Answer from the drawing. Dimensions are ordinates in mm from the lowest x, y and z of the part. A direction names the side the tool comes from. Coordinates: 2 decimals unless noted, no trailing zeros. Write each loop counter-clockwise with the first axis right and the second up, starting at its lowest first coordinate (ties: lowest second). Pieces come first, ordered by that corner, then holes. Notation, with made-up numbers: (-40, 19) - (-23, 19) arc R24 cw to (-23, 53) - close; hole circle Ø10 at (82.5, -30). An arc over 180 degrees is marked (long way). Return JSON: item names as keys, results as strings.
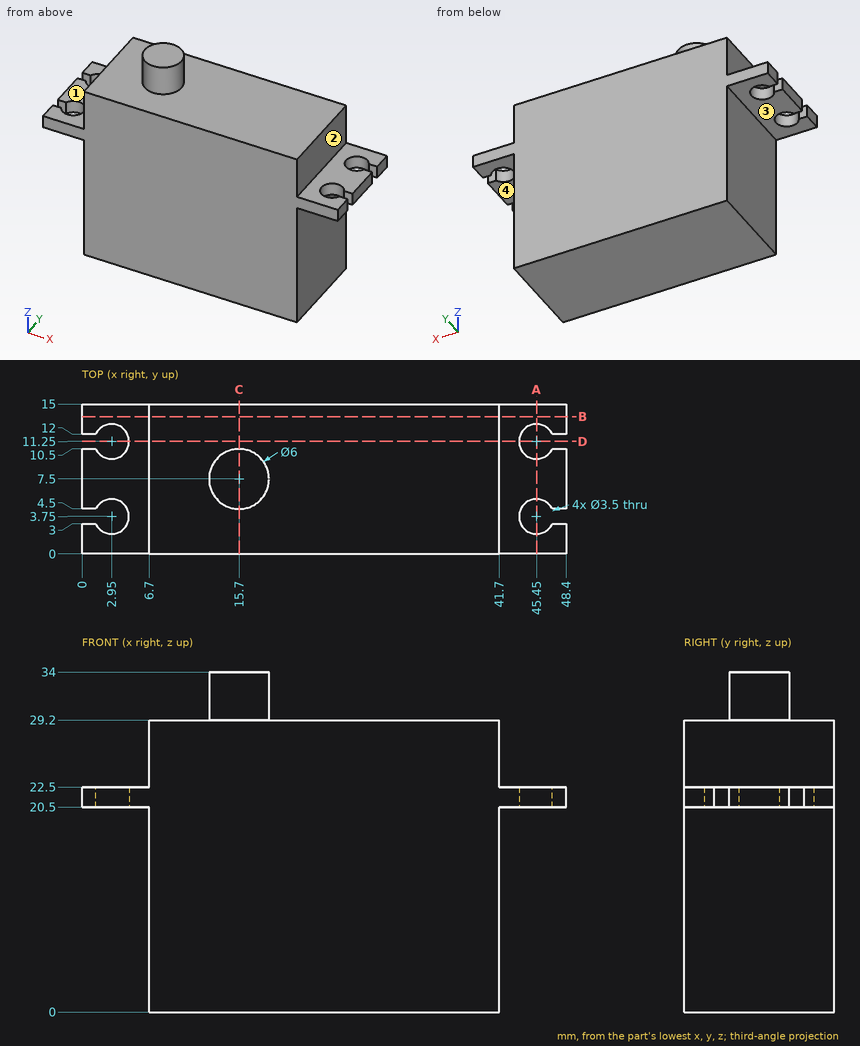
(1) A cutting plane is placed at D-D (y = 11.25). Determine the outline of the cut face in (x, z).
Answer:
{"outline": "(4.7, 20.5) - (6.7, 20.5) - (6.7, 0) - (41.7, 0) - (41.7, 20.5) - (43.7, 20.5) - (43.7, 22.5) - (41.7, 22.5) - (41.7, 29.2) - (6.7, 29.2) - (6.7, 22.5) - (4.7, 22.5) - close"}
(2) A cutting plane is placed at C-C (x = 15.7). Determine the outline of the cut face in (y, z).
Answer:
{"outline": "(0, 0) - (15, 0) - (15, 29.2) - (10.5, 29.2) - (10.5, 34) - (4.5, 34) - (4.5, 29.2) - (0, 29.2) - close"}
(3) Straight lines are drawn through the part: line 1 (Y direction, x = 2.95, z = 21.9); line 2 (Y direction, x = 45, z = 21); line 3 (Z direction, x = 43, y = 11.25). For each, find the intervals that lie inside material, in ascending order. Write a range as from..to.
Answer:
{"line 1": "0..2, 5.5..9.5, 13..15", "line 2": "0..2.06, 5.44..9.56, 12.94..15", "line 3": "20.5..22.5"}
(4) Flat-ended cylindrical pins translate along their axes: P1, Ø4, axis at x = 2.95, y = 3.75, coming from the +Z side; P2, Ø2, axis at y = 10.5, z = 27.5, coming from the +X side; P3, Ø4, axis at y = 3, z = 11.5, coming from the -X side. Find the tip coordinate at first contact, or state that the pin passes through.
Answer:
{"P1": "z = 22.5", "P2": "x = 41.7", "P3": "x = 6.7"}
(5) Which of the six approach directions +Z, -Z, +X, -X, +Y, -Y give full straight-line access (tool end or side, diameter ignored) to the marked faces 1, 2, 3 and 4?
Answer:
{"face 1": "+Z, -X, +Y, -Y", "face 2": "+Z, +X, +Y, -Y", "face 3": "-Z, -X, +Y, -Y", "face 4": "-Z, +X, +Y, -Y"}
(6) A cutting plane is placed at B-B (y = 13.75). Determine the outline of the cut face in (x, z).
Answer:
{"outline": "(0, 20.5) - (6.7, 20.5) - (6.7, 0) - (41.7, 0) - (41.7, 20.5) - (48.4, 20.5) - (48.4, 22.5) - (41.7, 22.5) - (41.7, 29.2) - (6.7, 29.2) - (6.7, 22.5) - (0, 22.5) - close"}
(7) A cutting plane is placed at A-A (x = 45.45). Determine the outline of the cut face in (y, z), and give its area (3 significant figures).
Answer:
{"outline": "(0, 20.5) - (2, 20.5) - (2, 22.5) - (0, 22.5) - close; (5.5, 20.5) - (9.5, 20.5) - (9.5, 22.5) - (5.5, 22.5) - close; (13, 20.5) - (15, 20.5) - (15, 22.5) - (13, 22.5) - close", "area": "16.0 mm²"}
